For this review, take the finished solid that the model builds, in its own axes (mm). Face numbers are marked on the shaded views. A direction names the side the tool comes from. Round coordinates to 2 decimals unless told otherwise and drop trailing zeros. Order: outer loops, then holes, each group sorted by start corner. A loop starts at its lowest first (then second) coordinate and runs counter-clockwise, first axis right, second up. Notation, with made-up numbers: (54.5, 13.5) -> (63.5, 13.5) arc R24 ccw to (63.5, 48.5) -> close; hole circle Ø11 at (81.25, 58). An arc over 180 degrees is marked (long way). Put each result on its own line as item: value. Start each with the question number.
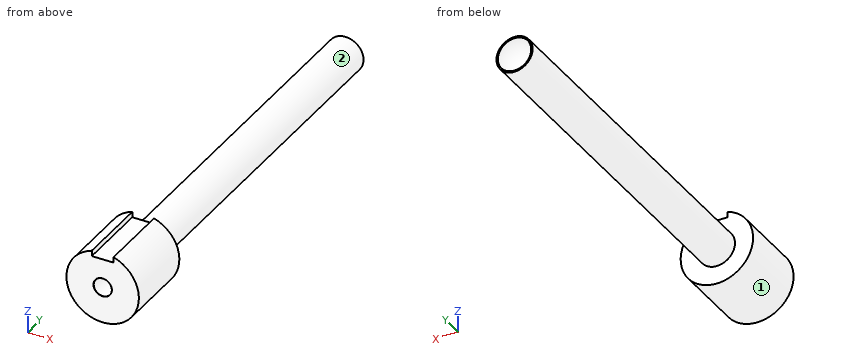
```python
from build123d import *

# Parameters (mm, degrees)
SKETCH1_R                             = 5
BOSS_EXTRUDE1_DEPTH                   = 10
SKETCH2_R                             = 2.5
BOSS_EXTRUDE2_DEPTH                   = 50
SKETCH9_W                             = 3
SKETCH9_H                             = 1.420897346
CUT_EXTRUDE2_DEPTH                    = 10
TAP_DRILL_FOR_M3X0_5_TAP2_D           = 2.5
TAP_DRILL_FOR_M3X0_5_TAP2_DEPTH       = 5
TAP_DRILL_FOR_M3X0_5_TAP2_CSINK_D     = 2.55
TAP_DRILL_FOR_M3X0_5_TAP2_CSINK_ANGLE = 90
TAP_DRILL_FOR_M3X0_5_TAP2_TIP         = 0.751075774


with BuildPart() as part:
    # Sketch1 → Boss-Extrude1 (new body)
    with BuildSketch(Plane(origin=(0, 0, 0), x_dir=(1, 0, 0), z_dir=(0, 1, 0))):
        with Locations(Location((0, 0, 0), (0, 0, 270))):
            Circle(SKETCH1_R)
    extrude(amount=BOSS_EXTRUDE1_DEPTH)

    # Sketch2 → Boss-Extrude2 (add)
    with BuildSketch(Plane(origin=(0, 10, 0), x_dir=(1, 0, 0), z_dir=(0, 1, 0))):
        with Locations(Location((0, 0, 0), (0, 0, 270))):
            Circle(SKETCH2_R)
    extrude(amount=BOSS_EXTRUDE2_DEPTH)

    # Sketch7 → Cut-Revolve1 (revolve, cut)
    with BuildSketch(Plane.XY):
        with BuildLine():
            Line((2.3, 60), (0, 60))
            Line((0, 60), (0, 57.7))
            ThreePointArc((0, 57.7), (1.626345597, 58.373654403), (2.3, 60))
        make_face()
    revolve(axis=Axis((0, 60, 0), (0, -1, 0)), mode=Mode.SUBTRACT)

    # Sketch9 → Cut-Extrude2 (cut)
    with BuildSketch(Plane.XZ):
        with Locations((0, 4.710448673)):
            Rectangle(SKETCH9_W, SKETCH9_H)
    extrude(amount=-CUT_EXTRUDE2_DEPTH, mode=Mode.SUBTRACT)

    # Tap Drill for M3x0.5 Tap2
    with Locations(Plane.XZ):
        with Locations((0, 0)):
            CounterSinkHole(TAP_DRILL_FOR_M3X0_5_TAP2_D / 2, TAP_DRILL_FOR_M3X0_5_TAP2_CSINK_D / 2, depth=TAP_DRILL_FOR_M3X0_5_TAP2_DEPTH, counter_sink_angle=TAP_DRILL_FOR_M3X0_5_TAP2_CSINK_ANGLE)
            with Locations((0, 0, -(TAP_DRILL_FOR_M3X0_5_TAP2_DEPTH + TAP_DRILL_FOR_M3X0_5_TAP2_TIP / 2))):  # 118° drill point
                Cone(0, TAP_DRILL_FOR_M3X0_5_TAP2_D / 2, TAP_DRILL_FOR_M3X0_5_TAP2_TIP, mode=Mode.SUBTRACT)


solid = part.part
```
Item 1: Tool access review of the marked faces 1 and 2: name each direction out of +Z, -Z, +X, -X, +Y, -Y from which nothing blocks a thin tool from reaching the whole face with its end or side.
Item 2: Consider section C-C, the plane z = 3.5. Write out the cut boundary in (x, y).
Item 3: Consider section B-B, the plane x = 4. Write out the cut boundary in (y, z).
Item 4: For L1, parallel to Z at x = 0, y = 2.8; L2, parallel to X at y = 3.35, z = 0; L3, parallel to Y at x = 3.25, z = 0, list the stretches that pass through material, from the lowest coordinate up.
Item 5: Insertion check: pin 1 Ø1.5 at (x, y) = (-0.5, 6) entering from +Z; pin 2 Ø1.5 at (y, z) = (45.5, 2) entering from +X; pin 3 Ø0.6 at (y, z) = (2.5, 4.5) entering from +X. Each pin has a flat end and moves straight along its axis. Give the tip position at first contact, or say it passes through.
Item 6: Consider section A-A, the plane y = 35.5. Write out the cut boundary in (x, z), plus the area to 3 significant figures.
Evaluation:
1. face 1: +Y, -Y
1. face 2: +Y
2. outline: (-3.57, 0) -> (3.57, 0) -> (3.57, 10) -> (-3.57, 10) -> close
3. outline: (0, -3) -> (10, -3) -> (10, 3) -> (0, 3) -> close
4. L1: z = -5 to -1.25, 1.25 to 4
4. L2: x = -5 to -1.25, 1.25 to 5
4. L3: y = 0 to 10
5. pin 1: stops at z = 4
5. pin 2: stops at x = 2.17
5. pin 3: stops at x = 2.71
6. outline: circle Ø5 at (0, 0)
6. area: 19.6 mm^2
